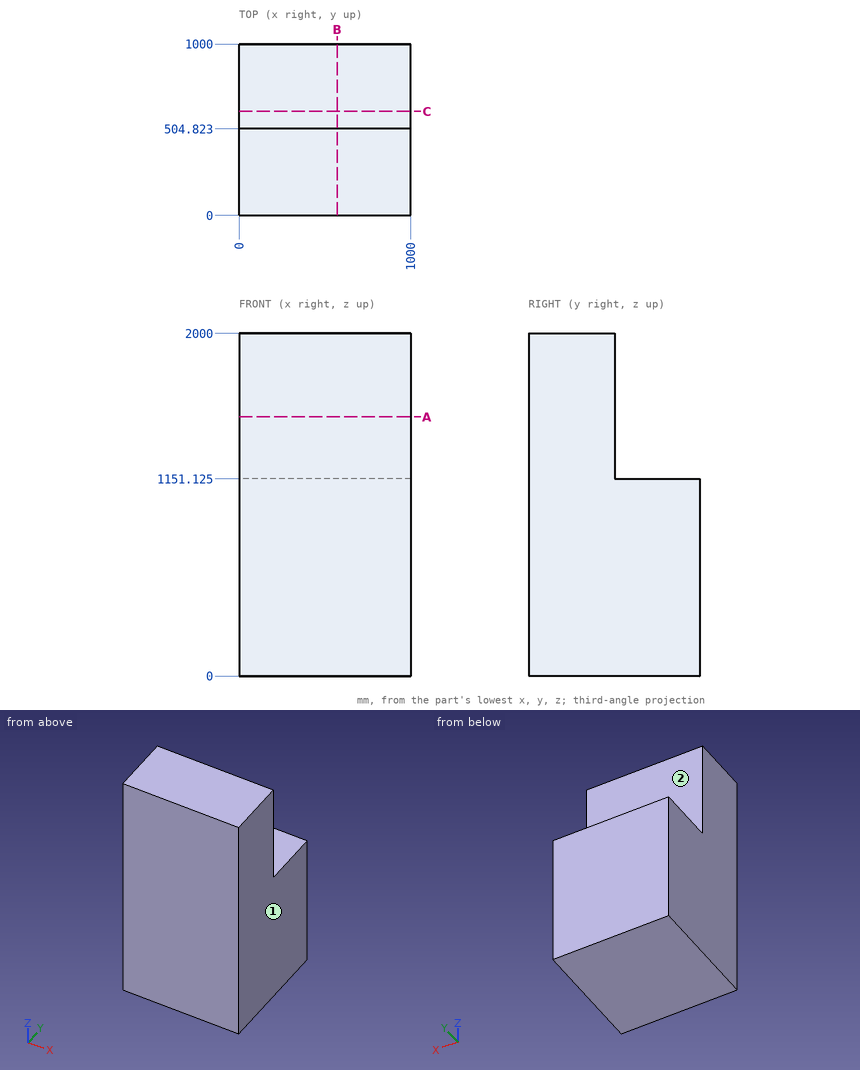
Answer from the drawing. Dimensions are ordinates in mm from the lowest x, y and z of the part. A direction names the side the tool comes from. Coordinates: 2 decimals unless noted, no trailing zeros. Order: outer loops, then holes, each group sorted by start corner. A loop starts at its lowest first (then second) coordinate and runs counter-clockwise, first axis right, second up. Notation, with made-up numbers: (2, 11) -> (55, 11) arc R32 ccw to (55, 50) -> close; hole circle Ø9 at (8.25, -32.5). An arc over 180 degrees is marked (long way). Answer as a JSON object with one key per item and string values.
1) Each of these flat-tipped pins is pushed along its axis until it touches: pin 1 (3 mm diameter, centred on y = 365, z = 1160, fed in from -X); pin 2 (1 mm diameter, centred on x = 561, y = 651.5, fed in from +Z) (1 decimal). Where does it stop, or does it pass through?
Model answer:
{"pin 1": "stops at x = 0", "pin 2": "stops at z = 1151.1"}
2) A cutting plane is placed at A-A, the plane z = 1512. Determine the outline of the cut face in (x, y).
Model answer:
{"outline": "(0, 0) -> (1000, 0) -> (1000, 504.82) -> (0, 504.82) -> close"}
3) Consider line 1 along Y through (x, z) = (540, 1167); line 2 along Z through (x, y) = (703, 627.5) (1 decimal). Determine where each line is inside the solid, lowest interval first. Write a range as from..to.
Model answer:
{"line 1": "y = 0..504.82", "line 2": "z = 0..1151.1"}
4) A cutting plane is placed at C-C, the plane y = 607. Determine the outline of the cut face in (x, z) (1 decimal).
Model answer:
{"outline": "(0, 0) -> (1000, 0) -> (1000, 1151.1) -> (0, 1151.1) -> close"}
5) A cutting plane is placed at B-B, the plane x = 572. Determine the outline of the cut face in (y, z) (1 decimal).
Model answer:
{"outline": "(0, 0) -> (1000, 0) -> (1000, 1151.1) -> (504.8, 1151.1) -> (504.8, 2000) -> (0, 2000) -> close"}
6) A tool of negligible diameter and unlimited length cuts with its end or side. For the marked faces 1 and 2, from which of +Z, -Z, +X, -X, +Y, -Y can it reach the whole face along a straight path? Write none if from no direction.
Model answer:
{"face 1": "+Z, -Z, +X, +Y, -Y", "face 2": "+Z, +X, -X, +Y"}
